Design review of the part built by this model. Coordinates are the model's own, in mm. A direction names the side the tool comes from. Coordinates: 2 decimals unless noted, no trailing zeros. Write each loop counter-clockwise with the first axis right and the second up, starting at its lowest first coordinate (ties: lowest second). Pieces come first, ordered by that corner, then holes.
Q1. Add section D-D, the plane z = -25.5. Give the boundary of the cut face in (x, y).
Q2. Add section C-C, the plane y = 17. Give the boundary of the cut face in (x, z).
Q3. Machinability: for faces 4 (the face through (-21, 0, -2)), 5 (the face through (-24, -23, -2)), which of the approach directions +Z, -Z, +X, -X, +Y, -Y give a long, thin tool a straight path to every point of the face, cutting with its end or side? Answer none if there is none.
Q4. Clearance check with a flat-ended pin moving along its axis: pin 1 Ø9 at (x, z) = (0, -115) entering from +Y. State where the tip first meets the part, or that it passes through.
Q5. Add section A-A, the plane x = 0. Give the boundary of the cut face in (y, z).
Q6. Add section B-B, the plane z = -115. Give the boundary of the cut face in (x, y), plus the area to 3 significant figures.
Q7. The part is to be moulded in two halves that separate along Y. For faces 1 (the face through (-23, 24, -2)), 2 (the face through (0, 23, -155)), 3 (the face through (21, 0, -2)), say which applies: +Y half, -Y half, draft (parallel to the pull), parting line (faces both ways), or undercut.
Q8. To check wall thickness, follow probe 1 along Z at (x, y) = (0, -22.85); probe 2 along Y at (x, z) = (12.5, -97.5). State the ranges of each line that lie inside material, in increasing order.
from build123d import *

# Parameters (mm, degrees)
TUBE_SQUARE_TS3X3X0_3125_3_DEPTH = 310
SKETCH12_R                       = 7.5
CUT_EXTRUDE1_DEPTH               = 165.772570533


with BuildPart() as part:
    # Sketch11 → Tube square TS3X3X0.3125(3) (new body)
    with BuildSketch(Plane(origin=(0, 0, -155), x_dir=(0, -1, 0), z_dir=(0, 0, 1))):
        with BuildLine():
            Line((-20, -25), (20, -25))
            ThreePointArc((20, -25), (23.535533906, -23.535533906), (25, -20))
            Line((25, -20), (25, 20))
            ThreePointArc((25, 20), (23.535533906, 23.535533906), (20, 25))
            Line((20, 25), (-20, 25))
            ThreePointArc((-20, 25), (-23.535533906, 23.535533906), (-25, 20))
            Line((-25, 20), (-25, -20))
            ThreePointArc((-25, -20), (-23.535533906, -23.535533906), (-20, -25))
        make_face()
        with BuildLine():
            Line((-20, -21), (20, -21))
            ThreePointArc((20, -21), (20.707106781, -20.707106781), (21, -20))
            Line((21, -20), (21, 20))
            ThreePointArc((21, 20), (20.707106781, 20.707106781), (20, 21))
            Line((20, 21), (-20, 21))
            ThreePointArc((-20, 21), (-20.707106781, 20.707106781), (-21, 20))
            Line((-21, 20), (-21, -20))
            ThreePointArc((-21, -20), (-20.707106781, -20.707106781), (-20, -21))
        make_face(mode=Mode.SUBTRACT)
    extrude(amount=TUBE_SQUARE_TS3X3X0_3125_3_DEPTH)

    # Sketch12 → Cut-Extrude1 (cut, through all)
    with BuildSketch(Plane(origin=(0, 25, 0), x_dir=(1, 0, 0), z_dir=(0, 1, 0))):
        with Locations(Location((0, 115, 0), (0, 0, 180))):
            Circle(SKETCH12_R)
    extrude(amount=-CUT_EXTRUDE1_DEPTH, mode=Mode.SUBTRACT)


solid = part.part
Here are the results:
1. outline: (-25, -20) arc R5 ccw to (-20, -25) - (20, -25) arc R5 ccw to (25, -20) - (25, 20) arc R5 ccw to (20, 25) - (-20, 25) arc R5 ccw to (-25, 20) - close; hole (-21, -20) arc R1 ccw to (-20, -21) - (20, -21) arc R1 ccw to (21, -20) - (21, 20) arc R1 ccw to (20, 21) - (-20, 21) arc R1 ccw to (-21, 20) - close
2. outline: (-25, -155) - (-21, -155) - (-21, 155) - (-25, 155) - close; (21, -155) - (25, -155) - (25, 155) - (21, 155) - close
3. face 4: +Z, -Z
3. face 5: +Z, -Z, -X, -Y
4. pin 1: passes through
5. outline: (-25, -155) - (-21, -155) - (-21, -122.5) - (-25, -122.5) - close; (-25, -107.5) - (-21, -107.5) - (-21, 155) - (-25, 155) - close; (21, -155) - (25, -155) - (25, -122.5) - (21, -122.5) - close; (21, -107.5) - (25, -107.5) - (25, 155) - (21, 155) - close
6. outline: (-25, -20) arc R5 ccw to (-20, -25) - (-7.5, -25) - (-7.5, -21) - (-20, -21) arc R1 cw to (-21, -20) - (-21, 20) arc R1 cw to (-20, 21) - (-7.5, 21) - (-7.5, 25) - (-20, 25) arc R5 ccw to (-25, 20) - close; (7.5, -25) - (20, -25) arc R5 ccw to (25, -20) - (25, 20) arc R5 ccw to (20, 25) - (7.5, 25) - (7.5, 21) - (20, 21) arc R1 cw to (21, 20) - (21, -20) arc R1 cw to (20, -21) - (7.5, -21) - close
6. area: 595 mm2
7. face 1: +Y half
7. face 2: draft
7. face 3: undercut
8. probe 1: z = -155 to -122.5, -107.5 to 155
8. probe 2: y = -25 to -21, 21 to 25
